Geometry: final body of the model. Coordinates: model frame, mm. Give positions to 0.01 mm unless a question says otherwise; leave off trailing zeros. Order: outer loops, then holes, each group sorted by start corner. A loop starts at its lowest first (then second) coordinate and runs counter-clockwise, first axis right, second up. Notation, with made-up numbers: M 37.25,88.5 L 92.25,88.5 A17 cw 92.25,105.5 Z; hole C 67,81.25 d11. An arc over 180 degrees is marked long. Use CSV: the item, a comma, the result in double quotes.
```python
from build123d import *

# Parameters (mm, degrees)
BOSS_EXTRUDE1_DEPTH = 18
SKETCH2_W           = 28.744942217
SKETCH2_H           = 2
SKETCH2_W_2         = 16.222921702
CUT_EXTRUDE1_DEPTH  = 3


with BuildPart() as part:
    # Sketch1 → Boss-Extrude1 (new body)
    with BuildSketch(Plane(origin=(0, 0, 0), x_dir=(1, 0, 0), z_dir=(0, 1, 0))):
        Polygon((171.5, 0), (0, 0), (0, -12), (183.5, -12), align=None)
        Polygon((0, 0), (-171.5, 0), (-183.5, -12), (0, -12), align=None)
    extrude(amount=BOSS_EXTRUDE1_DEPTH)

    # Sketch2 → Cut-Extrude1 (cut)
    with BuildSketch(Plane(origin=(0, 0, 0), x_dir=(-1, 0, 0), z_dir=(0, 0, -1))):
        Polygon((-148.243209669, 15), (-171.5, 15), (-171.5, 13), (-148.243209669, 13), (143.527924007, 13), (171.5, 13), (171.5, 15), (143.527924007, 15), align=None)
        with Locations((185.872471109, 14)):
            Rectangle(SKETCH2_W, SKETCH2_H)
        with Locations((-179.611460851, 14)):
            Rectangle(SKETCH2_W_2, SKETCH2_H)
    extrude(amount=-CUT_EXTRUDE1_DEPTH, mode=Mode.SUBTRACT)


solid = part.part
```
1. Section A-A, the plane x = -153.5. Return the cut outline in (y, z).
Answer:
outline,"M 0,0 L 13,0 L 13,3 L 15,3 L 15,0 L 18,0 L 18,12 L 0,12 Z"
2. Section C-C, the plane z = 7.5. Return the cut outline in (x, y).
Answer:
outline,"M -179,0 L 179,0 L 179,18 L -179,18 Z"
3. Pin query (flat end, axial travel): pin 1 Ø5 at (y, z) = (13, 6) entering from +X; pin 2 Ø6 at (y, z) = (9.5, 5) entering from -X. Return the tip coordinate at first contact, or that it passes through.
Answer:
pin 1,"x = 180"
pin 2,"x = -179.5"
4. Line query: line 1 (X direction, y = 10.75, z = 3); line 2 (Y direction, x = -0.5, z = 1); line 3 (Z direction, x = 153, y = 14). Output: solid intervals per line, ascending.
Answer:
line 1,"-174.5 to 174.5"
line 2,"0 to 13, 15 to 18"
line 3,"3 to 12"
5. Section B-B, the plane y = 10. Return the cut outline in (x, z).
Answer:
outline,"M -183.5,12 L -171.5,0 L 171.5,0 L 183.5,12 Z"
